CAD build for the part. Positions are in the model's coordinates, mm. A direction names the side the tool comes from. Coordinates: 2 decimals unless noted, no trailing zeros. Order: outer loops, then holes, each group sorted by start corner. A loop starts at its lowest first (then second) coordinate and runs counter-clockwise, first axis right, second up. Notation, with made-up numbers: M 82.25,56 L 107.25,56 A11 cw 107.25,70 Z; hole C -6.75,43 d4. An arc over 180 degrees is marked long. One line per item, written item: value.
from build123d import *

# Parameters (mm, degrees)
SKETCH_W     = 85
SKETCH_H     = 56
PAD_DEPTH    = 1.4
SKETCH001_R  = 1.25
POCKET_DEPTH = 204.998249
SKETCH002_W  = 17
SKETCH002_H  = 13.42
PAD001_DEPTH = 16
SKETCH003_W  = 21.3
SKETCH003_H  = 16
PAD002_DEPTH = 13.6
SKETCH004_W  = 51
SKETCH004_H  = 5
PAD003_DEPTH = 10.5
SKETCH005_W  = 51
SKETCH005_H  = 5
PAD004_DEPTH = 2.5


with BuildPart() as part:
    # Sketch → Pad (new body)
    with BuildSketch(Plane.XY):
        Rectangle(SKETCH_W, SKETCH_H)
    extrude(amount=PAD_DEPTH)

    # Sketch001 → Pocket (cut, through all)
    with BuildSketch(Plane.XY.offset(1.4)):
        with Locations((-39, 24.5)):
            Circle(SKETCH001_R)
        with Locations((19, 24.5)):
            Circle(SKETCH001_R)
    pocket = extrude(amount=-POCKET_DEPTH, mode=Mode.SUBTRACT)

    # Mirrored: Pocket across Sketch001 H_Axis
    add(pocket.mirror(Plane(origin=(0, 0, 1.4), x_dir=(0, 0, 1), z_dir=(0, 1, 0))), mode=Mode.SUBTRACT)

    # Sketch002 → Pad001 (new body)
    with BuildSketch(Plane.XY.offset(1.4)):
        with Locations((36, 19)):
            Rectangle(SKETCH002_W, SKETCH002_H)
        with Locations((36, 1)):
            Rectangle(SKETCH002_W, SKETCH002_H)
    extrude(amount=PAD001_DEPTH)

    # Sketch003 → Pad002 (new body)
    with BuildSketch(Plane.XY.offset(1.4)):
        with Locations((33.85, -17.75)):
            Rectangle(SKETCH003_W, SKETCH003_H)
    extrude(amount=PAD002_DEPTH)

    # Sketch004 → Pad003 (new body)
    with BuildSketch(Plane.XY.offset(1.4)):
        with Locations((-10, 24.5)):
            Rectangle(SKETCH004_W, SKETCH004_H)
    extrude(amount=PAD003_DEPTH)

    # Sketch005 → Pad004 (new body)
    with BuildSketch(Plane(origin=(0, 0, 0), x_dir=(1, 0, 0), z_dir=(0, 0, -1))):
        with Locations((-10, -24.5)):
            Rectangle(SKETCH005_W, SKETCH005_H)
    extrude(amount=PAD004_DEPTH)


solid = part.part
Q1. Slice it at C-C (z = 6.5). List the corners of the cut face in (x, y).
Recorded:
outline: M -35.5,22 L 15.5,22 L 15.5,27 L -35.5,27 Z; M 23.2,-25.75 L 44.5,-25.75 L 44.5,-9.75 L 23.2,-9.75 Z; M 27.5,-5.71 L 44.5,-5.71 L 44.5,7.71 L 27.5,7.71 Z; M 27.5,12.29 L 44.5,12.29 L 44.5,25.71 L 27.5,25.71 Z
Q2. Drill centre lines: line 1 along Y through (x, z) = (19, 1); line 2 along Y through (x, z) = (35.5, 8); line 3 along X through (y, z) = (-24.5, 0.4). Where is each one in solid material? Low to high.
Recorded:
line 1: y = -28 to -25.75, -23.25 to 23.25, 25.75 to 28
line 2: y = -25.75 to -9.75, -5.71 to 7.71, 12.29 to 25.71
line 3: x = -42.5 to -40.25, -37.75 to 17.75, 20.25 to 42.5
Q3. Slice it at D-D (y = 14.5). List the corners of the cut face in (x, z).
Recorded:
outline: M -42.5,0 L 42.5,0 L 42.5,1.4 L 44.5,1.4 L 44.5,17.4 L 27.5,17.4 L 27.5,1.4 L -42.5,1.4 Z
Q4. Mould opens along X. For faces 5 (the face through (20.155, -24.021, 0.71)), 6 (the face through (44.5, 19, 9)), 7 (the face through (34, -9.75, 8)) say: released by +X, released by -X, zero draft, split by the parting line, or undercut.
Recorded:
face 5: undercut
face 6: released by +X
face 7: zero draft
Q5. Slice it at A-A (x = -39). List the corners of the cut face in (y, z).
Recorded:
outline: M -28,0 L -25.75,0 L -25.75,1.4 L -28,1.4 Z; M -23.25,0 L 23.25,0 L 23.25,1.4 L -23.25,1.4 Z; M 25.75,0 L 28,0 L 28,1.4 L 25.75,1.4 Z
Q6. Which spindle directions (+Z, -Z, +X, -X, +Y, -Y) get a long thin tool onto all of the face, cutting with end or side? Do faces 1 (the face through (-35.5, 25, -1)), 2 (the face through (-10, 22, 7)), 3 (the face through (27.5, 19, 9)), 4 (the face through (36, -5.71, 9)). Say none if no direction does.
Recorded:
face 1: -Z, -X, +Y, -Y
face 2: +Z, -X, -Y
face 3: +Z, +Y
face 4: +Z, +X, -X
Q7. Slice it at B-B (y = -24.5). List the corners of the cut face in (x, z).
Recorded:
outline: M -42.5,0 L -40.25,0 L -40.25,1.4 L -42.5,1.4 Z; M -37.75,0 L 17.75,0 L 17.75,1.4 L -37.75,1.4 Z; M 20.25,0 L 42.5,0 L 42.5,1.4 L 44.5,1.4 L 44.5,15 L 23.2,15 L 23.2,1.4 L 20.25,1.4 Z
Q8. Pin check, flat tips, straight feed: pin 1 Ø12 at (x, y) = (-24.5, -7.5) entering from +Z; pin 2 Ø4 at (y, z) = (-14, 8.5) entering from -X; pin 3 Ø2 at (y, z) = (-0.5, 7) entering from -X. Stop position of each tip, or through.
Recorded:
pin 1: stops at z = 1.4
pin 2: stops at x = 23.2
pin 3: stops at x = 27.5
